```python
from build123d import *

# Parameters (mm, degrees)
CROQUIS1_R                 = 3
SALIENTE_EXTRUIR1_DEPTH    = 51
CORTAR_EXTRUIR1_DEPTH      = 311.888957589
CORTAR_EXTRUIR1_DEPTH_BACK = 311.888957589
CROQUIS2_W                 = 330
CROQUIS2_H                 = 30


with BuildPart() as part:
    # Croquis1 → Saliente-Extruir1 (new body)
    # profile 1 of 4: a face of its own
    with BuildSketch(Plane.XY):
        with BuildLine():
            Line((141.907724078, 74.393898239), (106.994802629, 58.391586929))
            ThreePointArc((106.994802629, 58.391586929), (116.540266028, 54.387158459), (115.408572004, 44.097815064))
            ThreePointArc((115.408572004, 44.097815064), (114.953536771, 43.612404014), (114.496565447, 43.128815181))
            Line((114.496565447, 43.128815181), (141.660745717, 55.579496794))
            ThreePointArc((141.660745717, 55.579496794), (163.715018222, 45.838294791), (185.769290727, 55.579496794))
            ThreePointArc((185.769290727, 55.579496794), (210.289811625, 39.891989826), (236.56917478, 52.411929606))
            ThreePointArc((236.56917478, 52.411929606), (262.563049751, 34.849044969), (290.598242925, 48.926132611))
            ThreePointArc((290.598242925, 48.926132611), (291.527530464, 63.45988081), (281.907724078, 74.393898239))
            add(Edge.make_bspline(
                [(141.907724078, 74.393898239), (211.705167047, 100.839206128), (281.907724078, 74.393898239)],
                knots=[0, 0, 0, 1, 1, 1], degree=2))
        make_face()
    # profile 2 of 4: a face of its own
    with BuildSketch(Plane.XY):
        with BuildLine():
            ThreePointArc((105.545350362, 57.727231572), (116.814352718, 53.541770784), (112.62889193, 42.272768428))
            Line((112.62889193, 42.272768428), (114.496565447, 43.128815181))
            ThreePointArc((114.496565447, 43.128815181), (114.953536771, 43.612404014), (115.408572004, 44.097815064))
            ThreePointArc((115.408572004, 44.097815064), (116.540266028, 54.387158459), (106.994802629, 58.391586929))
            Line((106.994802629, 58.391586929), (105.545350362, 57.727231572))
        make_face()
    # profile 3 of 4: a face of its own
    with BuildSketch(Plane.XY):
        with BuildLine():
            Line((-2.092318518, 8.391586929), (-3.541770784, 7.727231572))
            ThreePointArc((-3.541770784, 7.727231572), (-7.727231572, -3.541770784), (3.541770784, -7.727231572))
            Line((3.541770784, -7.727231572), (112.62889193, 42.272768428))
            ThreePointArc((112.62889193, 42.272768428), (116.814352718, 53.541770784), (105.545350362, 57.727231572))
            Line((105.545350362, 57.727231572), (104.095898096, 57.062876215))
            ThreePointArc((104.095898096, 57.062876215), (103.401090123, 56.516561913), (102.765670289, 55.902184936))
            ThreePointArc((102.765670289, 55.902184936), (55.876581472, 22.091691755), (-0.344694323, 8.641626802))
            ThreePointArc((-0.344694323, 8.641626802), (-1.224903213, 8.561316493), (-2.092318518, 8.391586929))
        make_face()
        Circle(CROQUIS1_R, mode=Mode.SUBTRACT)
        with Locations((109.087121146, 50)):
            Circle(CROQUIS1_R, mode=Mode.SUBTRACT)
    # profile 4 of 4: a face of its own
    with BuildSketch(Plane.XY):
        with BuildLine():
            ThreePointArc((3.541770784, -7.727231572), (-7.727231572, -3.541770784), (-3.541770784, 7.727231572))
            Line((-3.541770784, 7.727231572), (-2.092318518, 8.391586929))
            ThreePointArc((-2.092318518, 8.391586929), (-8.561316493, -1.224903213), (0.344694323, -8.641626802))
            ThreePointArc((0.344694323, -8.641626802), (62.478274911, 6.091677747), (114.496565447, 43.128815181))
            Line((114.496565447, 43.128815181), (112.62889193, 42.272768428))
            Line((112.62889193, 42.272768428), (3.541770784, -7.727231572))
        make_face()
    extrude(amount=SALIENTE_EXTRUIR1_DEPTH)

    # Croquis2 → Cortar-Extruir1 (cut, two sides: drawn at the far end of the back side and taken through both)
    with BuildSketch(Plane(origin=(-3.541770784, 7.727231572, 0), x_dir=(0.9090593428863096, 0.4166666666666667, 0), z_dir=(-0.41666666666666663, 0.9090593428863095, 0)).offset(-CORTAR_EXTRUIR1_DEPTH_BACK)):
        with Locations((-8.500249882, -25.5)):
            Rectangle(CROQUIS2_W, CROQUIS2_H)
    extrude(amount=CORTAR_EXTRUIR1_DEPTH + CORTAR_EXTRUIR1_DEPTH_BACK, mode=Mode.SUBTRACT)


solid = part.part
```
The model under review builds one solid part; all positions refer to its coordinate system, in mm. A direction names the side the tool comes from. Coordinates: 2 decimals unless noted, no trailing zeros. Write each loop counter-clockwise with the first axis right and the second up, starting at its lowest first coordinate (ties: lowest second). Pieces come first, ordered by that corner, then holes.
1) Machinability: for faces 4 (the face through (127.889, 49.267, 5.176)), 5 (the face through (-3, 0, 5)), 6 (the face through (144.184, 61.027, 25.71)), which of the approach directions +Z, -Z, +X, -X, +Y, -Y give a long, thin tool a straight path to every point of the face, cutting with its end or side? Answer none if there is none.
2) Clearance check with flat-ended pins moving along their axes: pin 1 Ø8 at (x, z) = (235, 12) entering from +Y; pin 2 Ø12 at (y, z) = (56.5, 18.5) entering from -X; pin 3 Ø1.5 at (y, z) = (24.5, 5.5) entering from -X. State where each tip first meets the part, or that it passes through.
3) We need section D-D on y = 29.5. State the section outline as (x, z) points, then the cut area to 3 significant figures.
4) The part is to be moulded in two halves that separate along Y. For faces 1 (the face through (175, 54, 51)), 2 (the face through (127.889, 49.267, 45.676)), 3 (the face through (106.88, 52.03, 45.68)), say which applies: pulls with the +Y half, pulls with the -Y half, needs draft (parallel to the pull), parting line crosses it, or undercut.
5) We need section A-A on y = 0. State the section outline as (x, z) points.
6) We need section C-C on z = 46. Count the separate pieces of the cut face and the enclosed holes in it, then the cut area to 3 significant figures.
7) To check wall thickness, follow probe 1 along Y at (x, z) = (0, 43.5); probe 2 along X at (y, z) = (50, 7); probe 3 along X at (y, z) = (45.5, 28). State the ranges of each line that lie inside material, in increasing order.
8) We need section B-B on x = 11.5. State the section outline as (y, z) points, then the cut area to 3 significant figures.
Answer list:
1. face 4: +Z, -Z, -Y
1. face 5: +Z, -Z
1. face 6: -X, -Y
2. pin 1: stops at y = 86.62
2. pin 2: stops at x = 143.51
2. pin 3: stops at x = 59.37
3. outline: (70, 0) - (99.92, 0) - (99.92, 10.5) - (70, 10.5) - close; (70, 40.5) - (99.92, 40.5) - (99.92, 51) - (70, 51) - close
3. area: 628 mm2
4. face 1: needs draft
4. face 2: pulls with the -Y half
4. face 3: undercut
5. outline: (-8.65, 0) - (-3, 0) - (-3, 10.5) - (-8.65, 10.5) - close; (-8.65, 40.5) - (-3, 40.5) - (-3, 51) - (-8.65, 51) - close; (3, 0) - (47.04, 0) - (47.04, 10.5) - (3, 10.5) - close; (3, 40.5) - (47.04, 40.5) - (47.04, 51) - (3, 51) - close
6. separate pieces: 1
6. enclosed holes: 2
6. area: 8,590 mm2
7. probe 1: y = -8.65 to -3, 3 to 8.66
7. probe 2: x = 96.94 to 106.09, 112.09 to 129.49, 148.52 to 178.91, 189.66 to 234.66, 237.86 to 291.08
7. probe 3: x = 194.62 to 229.7, 241.1 to 288.02
8. outline: (-7.82, 0) - (9.59, 0) - (9.59, 10.5) - (-7.82, 10.5) - close; (-7.82, 40.5) - (9.59, 40.5) - (9.59, 51) - (-7.82, 51) - close
8. area: 366 mm2
